Check sheet for the modelled part. Datum: model origin and axes. Units: mm. A direction names the side the tool comes from. Coordinates: 2 decimals unless noted, no trailing zeros. Loops run counter-clockwise (first coordinate to the right, second up) from the corner with the lowest first, then second, coordinate; pieces in that order, holes last.
```python
from build123d import *

# Parameters (mm, degrees)
SKETCH_2_W          = 10
SKETCH_2_H          = 88
EXTRUDE_1_DEPTH     = 16
EXTRUDE_1_2_DEPTH   = 16
SKETCH_3_W          = 10
SKETCH_3_H          = 20
EXTRUDE_2_DEPTH     = 158
SKETCH_4_R          = 10
EXTRUDE_3_DEPTH     = 124.5
SKETCH_5_R          = 2.2
CUT_EXTRUDE_1_DEPTH = 126
EXTRUDE_4_DEPTH     = 10
EXTRUDE_5_DEPTH     = 10


with BuildPart() as part:
    # Sketch 2 → Extrude 1 (new body)
    with BuildSketch(Plane(origin=(0, 0, 0), x_dir=(1, 0, 0), z_dir=(0, 1, 0))):
        with Locations((-57.25, 0)):
            Rectangle(SKETCH_2_W, SKETCH_2_H)
    extrude(amount=EXTRUDE_1_DEPTH)



with BuildPart() as body_2:
    # Sketch 2 → Extrude 1 2 (new body)
    with BuildSketch(Plane(origin=(0, 0, 0), x_dir=(1, 0, 0), z_dir=(0, 1, 0))):
        with Locations((57.25, 0)):
            Rectangle(SKETCH_2_W, SKETCH_2_H)
    extrude(amount=EXTRUDE_1_2_DEPTH)


with BuildPart() as part_1:
    add(part.part)

    add(body_2.part)  # Extrude 2 merges body 2
    # Sketch 3 → Extrude 2 (add)
    with BuildSketch(Plane(origin=(0, 16, 0), x_dir=(1, 0, 0), z_dir=(0, 1, 0))):
        with Locations((-57.25, 0)):
            Rectangle(SKETCH_3_W, SKETCH_3_H)
        with Locations((57.25, 0)):
            Rectangle(SKETCH_3_W, SKETCH_3_H)
    extrude(amount=EXTRUDE_2_DEPTH)

    # Sketch 4 → Extrude 3 (add)
    with BuildSketch(Plane.ZY.offset(62.25)):
        with Locations((0, 174)):
            Circle(SKETCH_4_R)
    extrude(amount=-EXTRUDE_3_DEPTH)

    # Sketch 5 → Cut-Extrude 1 (cut)
    with BuildSketch(Plane.ZY.offset(62.25)):
        with Locations((0, 8)):
            Circle(SKETCH_5_R)
        with Locations((-34, 8)):
            Circle(SKETCH_5_R)
        with Locations((34, 8)):
            Circle(SKETCH_5_R)
    extrude(amount=-CUT_EXTRUDE_1_DEPTH, mode=Mode.SUBTRACT)

    # Sketch 6 → Extrude 4 (add)
    with BuildSketch(Plane.ZY.offset(62.25)):
        Polygon((-44, 16), (-10, 95), (-10, 55.5), (-27, 16), align=None)
        Polygon((44, 16), (10, 95), (10, 55.5), (27, 16), align=None)
    extrude(amount=-EXTRUDE_4_DEPTH)

    # Sketch 7 → Extrude 5 (add)
    with BuildSketch(Plane(origin=(62.25, 0, 0), x_dir=(0, 0, -1), z_dir=(1, 0, 0))):
        Polygon((-44, 16), (-10, 95), (-10, 55.5), (-27, 16), align=None)
        Polygon((44, 16), (10, 95), (10, 55.5), (27, 16), align=None)
    extrude(amount=-EXTRUDE_5_DEPTH)


solid = part_1.part
```
1) Section check D-D on z = -19. Enter the section's corners in (x, y).
Answer sheet:
outline: (-62.25, 0) - (-52.25, 0) - (-52.25, 16) - (-62.25, 16) - close; (-62.25, 34.59) - (-52.25, 34.59) - (-52.25, 74.09) - (-62.25, 74.09) - close; (52.25, 0) - (62.25, 0) - (62.25, 16) - (52.25, 16) - close; (52.25, 34.59) - (62.25, 34.59) - (62.25, 74.09) - (52.25, 74.09) - close
2) Section check B-B on z = 0. Enter the section's corners in (x, y).
Answer sheet:
outline: (-62.25, 0) - (-52.25, 0) - (-52.25, 5.8) - (-62.25, 5.8) - close; (-62.25, 10.2) - (-52.25, 10.2) - (-52.25, 164) - (52.25, 164) - (52.25, 10.2) - (62.25, 10.2) - (62.25, 184) - (-62.25, 184) - close; (52.25, 0) - (62.25, 0) - (62.25, 5.8) - (52.25, 5.8) - close
3) Scan lines: line 1 (Y direction, x = 57.75, z = 0); line 2 (X direction, y = 165, z = 7.5); line 3 (Y direction, x = -54, z = -34). Record each from-to range of solid material in increasing order.
Answer sheet:
line 1: y = 0 to 5.8, 10.2 to 184
line 2: x = -62.25 to -52.25, 52.25 to 62.25
line 3: y = 0 to 5.8, 10.2 to 39.24
4) Section check A-A on y = 138. Enter the section's corners in (x, z), plus the area to 3 significant figures.
Answer sheet:
outline: (-62.25, -10) - (-52.25, -10) - (-52.25, 10) - (-62.25, 10) - close; (52.25, -10) - (62.25, -10) - (62.25, 10) - (52.25, 10) - close
area: 400 mm2
5) Depth check by flat-ended pin: pin 1 (7 mm diameter, centred on y = 8, z = 0, fed in from -X); pin 2 (5 mm diameter, centred on x = -57, y = 117.5, fed in from -Z); pin 3 (11 mm diameter, centred on x = -56.5, y = 32.5, fed in from -Z); pin 4 (11 mm diameter, centred on x = -57, y = 151, fed in from +Z). Enter the tip coordinate at first touch or a pass-through.
Answer sheet:
pin 1: stops at x = -62.25
pin 2: stops at z = -10
pin 3: stops at z = -39.27
pin 4: stops at z = 10
6) Mould release check, pull along Z, two halves, no side actions. Record for faces 1 (the cylindrical face through (-0.871, 183.915, -1.302)), 2 (the flat face through (57, 134, 10)), 3 (the flat face through (57, 35, -10)): +Z half, -Z half, draft (parallel to the pull), parting line (faces both ways), or undercut.
Answer sheet:
face 1: parting line
face 2: +Z half
face 3: undercut
7) Section check C-C on y = 8. Give the number of separate pieces and of enclosed holes in the cut face, plus the area to 3 significant figures.
Answer sheet:
separate pieces: 8
enclosed holes: 0
area: 1,500 mm2
8) Set-up check for faces 4 (the flat face through (57, 16, -19)), 5 (the flat face through (-57, 134, 10)), 6 (the flat face through (-57, 134, -10)): record each of +Z, -Z, +X, -X, +Y, -Y from which the full face is reachable in a straight line by a thin tool's end or side.
Answer sheet:
face 4: +X, -X
face 5: +Z, +X, -X, +Y
face 6: -Z, +X, -X, +Y
